```python
from build123d import *

# Parameters (mm, degrees)
SKETCH1_W           = 145
SKETCH1_H           = 21.8
BOSS_EXTRUDE1_DEPTH = 3.8
SKETCH2_W           = 12
SKETCH2_H           = 11
CUT_EXTRUDE1_DEPTH  = 147.678832829
SKETCH3_R           = 2.25
CUT_EXTRUDE2_DEPTH  = 147.678832829
SKETCH4_R           = 0.5
CUT_EXTRUDE3_DEPTH  = 147.678832829
SKETCH5_W           = 10
SKETCH5_H           = 3.8
BOSS_EXTRUDE2_DEPTH = 3.8
LPATTERN1_COUNT     = 4
LPATTERN1_PITCH     = 20
LPATTERN1_COL_COUNT = 4
LPATTERN1_COL_PITCH = 20
SKETCH6_W           = 145
SKETCH6_H           = 3
BOSS_EXTRUDE3_DEPTH = 3.8
SKETCH8_W           = 10
SKETCH8_H           = 3.8
CUT_EXTRUDE4_DEPTH  = 148.842483745
SKETCH9_W           = 3.8
SKETCH9_H           = 5
CUT_EXTRUDE5_DEPTH  = 148.842483745
SKETCH10_W          = 12.8
SKETCH10_H          = 3
CUT_EXTRUDE6_DEPTH  = 148.842483745
SKETCH11_W          = 10
SKETCH11_H          = 3.8
BOSS_EXTRUDE4_DEPTH = 3.8
LPATTERN2_COUNT     = 3
LPATTERN2_PITCH     = 20
SKETCH12_W          = 10
SKETCH12_H          = 3.8
BOSS_EXTRUDE5_DEPTH = 3.8
LPATTERN3_COUNT     = 4
LPATTERN3_PITCH     = 20
SKETCH13_W          = 6
SKETCH13_H          = 3
CUT_EXTRUDE7_DEPTH  = 148.842483745
FILLET1_R           = 1


with BuildPart() as part:
    # Sketch1 → Boss-Extrude1 (new body)
    with BuildSketch(Plane(origin=(0, 0, 0), x_dir=(1, 0, 0), z_dir=(0, 1, 0))):
        with Locations((72.5, -10.9)):
            Rectangle(SKETCH1_W, SKETCH1_H)
    extrude(amount=BOSS_EXTRUDE1_DEPTH)

    # Sketch2 → Cut-Extrude1 (cut, through all)
    with BuildSketch(Plane(origin=(0, 3.8, 0), x_dir=(1, 0, 0), z_dir=(0, 1, 0))):
        with Locations((72.5, -10)):
            Rectangle(SKETCH2_W, SKETCH2_H)
    extrude(amount=-CUT_EXTRUDE1_DEPTH, mode=Mode.SUBTRACT)

    # Sketch3 → Cut-Extrude2 (cut, through all)
    with BuildSketch(Plane(origin=(0, 3.8, 0), x_dir=(1, 0, 0), z_dir=(0, 1, 0))):
        with Locations(Location((42, -4, 0), (0, 0, 270))):
            Circle(SKETCH3_R)
        with Locations(Location((135, -4, 0), (0, 0, 270))):
            Circle(SKETCH3_R)
    extrude(amount=-CUT_EXTRUDE2_DEPTH, mode=Mode.SUBTRACT)

    # Sketch4 → Cut-Extrude3 (cut, through all)
    with BuildSketch(Plane(origin=(0, 3.8, 0), x_dir=(1, 0, 0), z_dir=(0, 1, 0))):
        with BuildLine():
            Line((98.5, -7.8), (98.5, -16.8))
            Line((98.5, -16.8), (105.5, -16.8))
            ThreePointArc((105.5, -16.8), (110, -12.300000006), (105.500000011, -7.8))
            Line((105.500000011, -7.8), (98.5, -7.8))
        make_face()
        with Locations(Location((96.75, -12.3, 0), (0, 0, 270))):
            Circle(SKETCH4_R)
        with Locations(Location((111.75, -12.3, 0), (0, 0, 270))):
            Circle(SKETCH4_R)
    extrude(amount=-CUT_EXTRUDE3_DEPTH, mode=Mode.SUBTRACT)

    # Sketch5 → Boss-Extrude2 (add, through all)
    with BuildSketch(Plane(origin=(0, 3.8, 0), x_dir=(1, 0, 0), z_dir=(0, 1, 0))):
        with Locations((72.5, -23.7)):
            Rectangle(SKETCH5_W, SKETCH5_H)
    boss_extrude2 = extrude(amount=-BOSS_EXTRUDE2_DEPTH)

    # LPattern1: Boss-Extrude2 ×4
    with Locations(*[(-i * LPATTERN1_PITCH, 0, 0) for i in range(1, LPATTERN1_COUNT)]):
        add(boss_extrude2)

    # LPattern1 col: Boss-Extrude2 ×4
    with Locations(*[(i * LPATTERN1_COL_PITCH, 0, 0) for i in range(1, LPATTERN1_COL_COUNT)]):
        add(boss_extrude2)

    # Sketch6 → Boss-Extrude3 (add, through all)
    with BuildSketch(Plane(origin=(0, 3.8, 0), x_dir=(1, 0, 0), z_dir=(0, 1, 0))):
        with Locations((72.5, -27.1)):
            Rectangle(SKETCH6_W, SKETCH6_H)
    extrude(amount=-BOSS_EXTRUDE3_DEPTH)

    # Sketch8 → Cut-Extrude4 (cut, through all)
    with BuildSketch(Plane(origin=(0, 0, 0), x_dir=(-1, 0, 0), z_dir=(0, -1, 0))):
        with Locations((-12.5, -23.7)):
            Rectangle(SKETCH8_W, SKETCH8_H)
        with Locations((-132.5, -23.7)):
            Rectangle(SKETCH8_W, SKETCH8_H)
    extrude(amount=-CUT_EXTRUDE4_DEPTH, mode=Mode.SUBTRACT)

    # Sketch9 → Cut-Extrude5 (cut, through all)
    with BuildSketch(Plane(origin=(0, 3.8, 0), x_dir=(1, 0, 0), z_dir=(0, 1, 0))):
        with Locations((1.9, -15.5)):
            Rectangle(SKETCH9_W, SKETCH9_H)
        with Locations((1.9, -5.5)):
            Rectangle(SKETCH9_W, SKETCH9_H)
        with Locations((143.1, -15.5)):
            Rectangle(SKETCH9_W, SKETCH9_H)
        with Locations((143.1, -5.5)):
            Rectangle(SKETCH9_W, SKETCH9_H)
    extrude(amount=-CUT_EXTRUDE5_DEPTH, mode=Mode.SUBTRACT)

    # Sketch10 → Cut-Extrude6 (cut, through all)
    with BuildSketch(Plane(origin=(0, 0, 0), x_dir=(-1, 0, 0), z_dir=(0, -1, 0))):
        with Locations((-6.4, -27.1)):
            Rectangle(SKETCH10_W, SKETCH10_H)
        with Locations((-138.6, -27.1)):
            Rectangle(SKETCH10_W, SKETCH10_H)
    extrude(amount=-CUT_EXTRUDE6_DEPTH, mode=Mode.SUBTRACT)

    # Sketch11 → Boss-Extrude4 (add, through all)
    with BuildSketch(Plane(origin=(0, 0, 0), x_dir=(-1, 0, 0), z_dir=(0, -1, 0))):
        with Locations((-5, 1.9)):
            Rectangle(SKETCH11_W, SKETCH11_H)
    boss_extrude4 = extrude(amount=-BOSS_EXTRUDE4_DEPTH)

    # LPattern2: Boss-Extrude4 ×3
    with Locations(*[(i * LPATTERN2_PITCH, 0, 0) for i in range(1, LPATTERN2_COUNT)]):
        add(boss_extrude4)

    # Sketch12 → Boss-Extrude5 (add, through all)
    with BuildSketch(Plane(origin=(0, 0, 0), x_dir=(-1, 0, 0), z_dir=(0, -1, 0))):
        with Locations((-140, 1.9)):
            Rectangle(SKETCH12_W, SKETCH12_H)
    boss_extrude5 = extrude(amount=-BOSS_EXTRUDE5_DEPTH)

    # LPattern3: Boss-Extrude5 ×4
    with Locations(*[(-i * LPATTERN3_PITCH, 0, 0) for i in range(1, LPATTERN3_COUNT)]):
        add(boss_extrude5)

    # Sketch13 → Cut-Extrude7 (cut, through all)
    with BuildSketch(Plane(origin=(0, 3.8, 0), x_dir=(1, 0, 0), z_dir=(0, 1, 0))):
        with Locations((135, -4)):
            Rectangle(SKETCH13_W, SKETCH13_H)
    extrude(amount=-CUT_EXTRUDE7_DEPTH, mode=Mode.SUBTRACT)

    # Fillet1
    fillet1_edges = [part.edges().sort_by_distance(p)[0] for p in [
        (138, 1.9, 5.5),
        (132, 1.9, 2.5),
        (138, 1.9, 2.5),
        (132, 1.9, 5.5),
    ]]
    fillet(fillet1_edges, radius=FILLET1_R)


solid = part.part
```
Build history of the part. All positions in model axes, mm. A direction names the side the tool comes from. Round coordinates to 2 decimals unless told otherwise and drop trailing zeros. Write each loop counter-clockwise with the first axis right and the second up, starting at its lowest first coordinate (ties: lowest second). Pieces come first, ordered by that corner, then holes.
1) Pin check, flat tips, straight feed: pin 1 (2 mm diameter, centred on x = 100.5, z = 13, fed in from +Y); pin 2 (1.9 mm diameter, centred on x = 72.5, y = 2, fed in from -Z); pin 3 (1.9 mm diameter, centred on y = 1, z = 23, fed in from -X). Stop position of each tip, or through.
2) Band-saw the part on C-C, the plane y = 0.8. Give the number of separate pieces and of enclosed holes in the cut face, and give its area (3 significant figures).
3) Drill centre lines: probe 1 along X at (y, z) = (2.8, 12.3); probe 2 along X at (y, z) = (3.55, 22); probe 3 along Z at (x, y) = (38, 0.8). Where is each one in solid material? Low to high.
4) Band-saw the part on B-B, the plane x = 42. List the corners of the cut face in (y, z), and give its area (3 significant figures).
5) 3-axis set-ups, long thin cutter, end or side, ignore diameter. For faces 1 (the flat face through (2, 2, 13)), 2 (the flat face through (102, 2, 25.6)), 3 (the flat face through (130, 2, 0)): which of +Z, -Z, +X, -X, +Y, -Y reach the whole face in a straight line?
6) Mould opens along X. For faces 4 (the flat face through (141.2, 2, 16)), 5 (the flat face through (0, 2, 0)), 6 (the flat face through (143, 2, 18)), 7 (the flat face through (62, 2, 21.8)) say: +X half, -X half, draft (parallel to the pull), parting line (faces both ways), or undercut.
7) Band-saw the part on A-A, the plane x = 130.5. List the corners of the cut face in (y, z), and give its area (3 significant figures).
Ans:
1. pin 1: passes through
1. pin 2: stops at z = 0
1. pin 3: stops at x = 27.5
2. separate pieces: 1
2. enclosed holes: 10
2. area: 3,630 mm2
3. probe 1: x = 0 to 66.5, 78.5 to 96.25, 97.25 to 98.5, 110 to 111.25, 112.25 to 145
3. probe 2: x = 27.5 to 37.5, 47.5 to 57.5, 67.5 to 77.5, 87.5 to 97.5, 107.5 to 117.5
3. probe 3: z = 0 to 21.8, 25.6 to 28.6
4. outline: (0, -3.8) - (3.8, -3.8) - (3.8, 1.75) - (0, 1.75) - close; (0, 6.25) - (3.8, 6.25) - (3.8, 21.8) - (0, 21.8) - close; (0, 25.6) - (3.8, 25.6) - (3.8, 28.6) - (0, 28.6) - close
4. area: 91.6 mm2
5. face 1: -X, +Y, -Y
5. face 2: +Y, -Y
5. face 3: -Z, +Y, -Y
6. face 4: +X half
6. face 5: -X half
6. face 6: draft
6. face 7: undercut
7. outline: (0, 0) - (3.8, 0) - (3.8, 21.8) - (0, 21.8) - close; (0, 25.6) - (3.8, 25.6) - (3.8, 28.6) - (0, 28.6) - close
7. area: 94.2 mm2
